Source: CAD feature listing. Evaluate the final solid. Frame: model axes, mm. Round coordinates to 2 decimals unless told otherwise and drop trailing zeros. Order: outer loops, then holes, each group sorted by start corner. A loop starts at its lowest first (then second) coordinate and runs counter-clockwise, first axis right, second up. Notation, with made-up numbers: (1, 40) -> (39, 40) arc R16 cw to (39, 66) -> close; hole circle Ø9 at (17, 1.5). An arc over 180 degrees is marked (long way). Answer as CSV lines item,"result". Start each with the question number.
(1) Section query A-A (y = -5). Output: boundary loops of the cut face in (x, z), plus the area to 3 significant figures.
(2) Section query B-B (x = -7). Output: boundary loops of the cut face in (y, z) (3 decimals).
(3) Line query: line 1 along Z through (x, y) = (-21, -7.5); line 2 along Y through (x, z) = (0, 411) (3 decimals). Output: solid intervals per line, ascending. Write a range as from..to.
(4) Section query C-C (z = 409.5). Output: boundary loops of the cut face in (x, y) (3 decimals), plus the area to 3 significant figures.
(5) Contact query for flat-ended pins moving along their axis: P1, Ø5, axis at x = 0.5, y = -5.5, coming from the -Z side; P2, Ø15, axis at x = -9, z = 404.5, coming from the -Y side. Output: stop coordinate, or through.
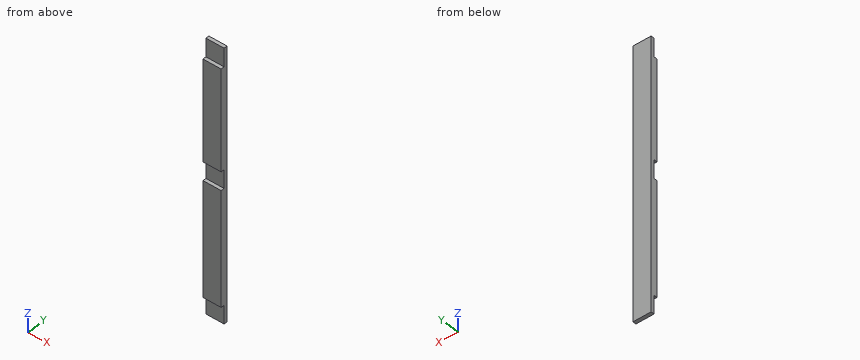
```python
from build123d import *

# Parameters (mm, degrees)
F0_W     = 50.8
F0_H     = 19.05
F1_DEPTH = 749.3
F2_W     = 122.435573
F2_H     = 50.8
F2_W_2   = 93.867282
F2_W_3   = 343.160421
F3_DEPTH = 25.4


with BuildPart() as f1:
    # F0 (on Top) → F1 (new body)
    with BuildSketch(Plane.XY):
        Rectangle(F0_W, F0_H)
    extrude(amount=F1_DEPTH)

    # F2 (on Front) → F3 (cut)
    with BuildSketch(Plane.XZ):
        with Locations((22.446524, 25.4)):
            Rectangle(F2_W, F2_H)
        with Locations((2.720783, 393.7)):
            Rectangle(F2_W_2, F2_H)
        with Locations((-38.781822, 723.9)):
            Rectangle(F2_W_3, F2_H)
    extrude(amount=F3_DEPTH, mode=Mode.SUBTRACT)


solid = f1.part
```
Answer block:
1,outline,"(-25.4, 50.8) -> (25.4, 50.8) -> (25.4, 368.3) -> (-25.4, 368.3) -> close; (-25.4, 419.1) -> (25.4, 419.1) -> (25.4, 698.5) -> (-25.4, 698.5) -> close"
1,area,"30,300 mm2"
2,outline,"(-9.525, 50.8) -> (0, 50.8) -> (0, 0) -> (9.525, 0) -> (9.525, 749.3) -> (0, 749.3) -> (0, 698.5) -> (-9.525, 698.5) -> (-9.525, 419.1) -> (0, 419.1) -> (0, 368.3) -> (-9.525, 368.3) -> close"
3,line 1,"50.8..368.3, 419.1..698.5"
3,line 2,"0..9.525"
4,outline,"(-25.4, 0) -> (25.4, 0) -> (25.4, 9.525) -> (-25.4, 9.525) -> close"
4,area,"484 mm2"
5,P1,"z = 50.8"
5,P2,"y = 0"
